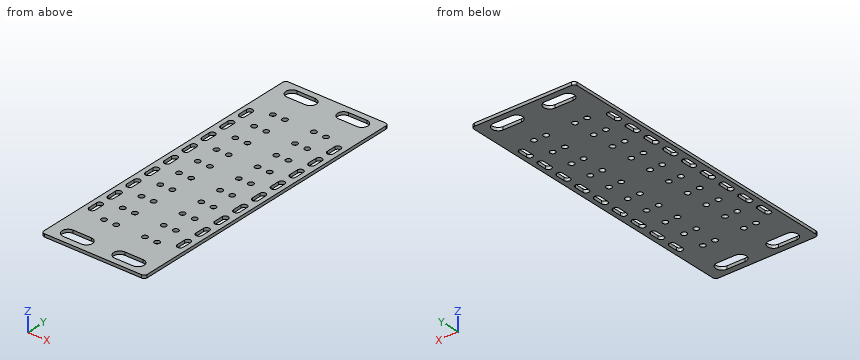
```python
from build123d import *

# Parameters (mm, degrees)
ESBO_O1_W             = 68
ESBO_O1_H             = 195
FLANGE_BASE1_DEPTH    = 2
FILETE1_R             = 2
ESBO_O2_R             = 1.75
CORTE_EXTRUS_O1_DEPTH = 10


# Sheet-metal steps are written as plain solids
with BuildPart() as part:
    # Esboço1 → Flange-base1 (new body)
    with BuildSketch(Plane.XY):
        with Locations((34, 97.5)):
            Rectangle(ESBO_O1_W, ESBO_O1_H)
    extrude(amount=-FLANGE_BASE1_DEPTH)

    # Filete1
    filete1_edges = [part.edges().sort_by_distance(p)[0] for p in [
        (0, 195, -1),
        (68, 195, -1),
        (68, 0, -1),
        (0, 0, -1),
    ]]
    fillet(filete1_edges, radius=FILETE1_R)

    # Esboço2 → Corte-extrusão1 (cut)
    with BuildSketch(Plane.XY):
        with Locations((16.5, 165)):
            Circle(ESBO_O2_R)
        with Locations((24.5, 165)):
            Circle(ESBO_O2_R)
        with Locations((43.5, 165)):
            Circle(ESBO_O2_R)
        with Locations((51.5, 165)):
            Circle(ESBO_O2_R)
        with Locations((43.5, 150)):
            Circle(ESBO_O2_R)
        with Locations((51.5, 150)):
            Circle(ESBO_O2_R)
        with Locations((43.5, 135)):
            Circle(ESBO_O2_R)
        with Locations((51.5, 135)):
            Circle(ESBO_O2_R)
        with Locations((43.5, 120)):
            Circle(ESBO_O2_R)
        with Locations((51.5, 120)):
            Circle(ESBO_O2_R)
        with Locations((43.5, 105)):
            Circle(ESBO_O2_R)
        with Locations((51.5, 105)):
            Circle(ESBO_O2_R)
        with Locations((16.5, 150)):
            Circle(ESBO_O2_R)
        with Locations((24.5, 150)):
            Circle(ESBO_O2_R)
        with Locations((16.5, 135)):
            Circle(ESBO_O2_R)
        with Locations((24.5, 135)):
            Circle(ESBO_O2_R)
        with Locations((16.5, 120)):
            Circle(ESBO_O2_R)
        with Locations((24.5, 120)):
            Circle(ESBO_O2_R)
        with Locations((16.5, 105)):
            Circle(ESBO_O2_R)
        with Locations((24.5, 105)):
            Circle(ESBO_O2_R)
        with Locations((16.5, 90)):
            Circle(ESBO_O2_R)
        with Locations((24.5, 90)):
            Circle(ESBO_O2_R)
        with Locations((43.5, 90)):
            Circle(ESBO_O2_R)
        with Locations((51.5, 90)):
            Circle(ESBO_O2_R)
        with Locations((16.5, 75)):
            Circle(ESBO_O2_R)
        with Locations((24.5, 75)):
            Circle(ESBO_O2_R)
        with Locations((43.5, 75)):
            Circle(ESBO_O2_R)
        with Locations((51.5, 75)):
            Circle(ESBO_O2_R)
        with Locations((16.5, 60)):
            Circle(ESBO_O2_R)
        with Locations((24.5, 60)):
            Circle(ESBO_O2_R)
        with Locations((43.5, 60)):
            Circle(ESBO_O2_R)
        with Locations((51.5, 60)):
            Circle(ESBO_O2_R)
        with Locations((16.5, 45)):
            Circle(ESBO_O2_R)
        with Locations((24.5, 45)):
            Circle(ESBO_O2_R)
        with Locations((43.5, 45)):
            Circle(ESBO_O2_R)
        with Locations((51.5, 45)):
            Circle(ESBO_O2_R)
        with Locations((16.5, 30)):
            Circle(ESBO_O2_R)
        with Locations((24.5, 30)):
            Circle(ESBO_O2_R)
        with Locations((43.5, 30)):
            Circle(ESBO_O2_R)
        with Locations((51.5, 30)):
            Circle(ESBO_O2_R)
        with BuildLine():
            Line((11, 191), (23, 191))
            ThreePointArc((23, 191), (27, 187), (23, 183))
            Line((23, 183), (11, 183))
            ThreePointArc((11, 183), (7, 187), (11, 191))
        make_face()
        with BuildLine():
            Line((57, 191), (45, 191))
            ThreePointArc((45, 191), (41, 187), (45, 183))
            Line((45, 183), (57, 183))
            ThreePointArc((57, 183), (61, 187), (57, 191))
        make_face()
        with BuildLine():
            Line((11, 4), (23, 4))
            ThreePointArc((23, 4), (27, 8), (23, 12))
            Line((23, 12), (11, 12))
            ThreePointArc((11, 12), (7, 8), (11, 4))
        make_face()
        with BuildLine():
            Line((57, 4), (45, 4))
            ThreePointArc((45, 4), (41, 8), (45, 12))
            Line((45, 12), (57, 12))
            ThreePointArc((57, 12), (61, 8), (57, 4))
        make_face()
        with BuildLine():
            Line((7, 160.5), (7, 154.5))
            ThreePointArc((7, 154.5), (5, 152.5), (3, 154.5))
            Line((3, 154.5), (3, 160.5))
            ThreePointArc((3, 160.5), (5, 162.5), (7, 160.5))
        make_face()
        with BuildLine():
            Line((65, 160.5), (65, 154.5))
            ThreePointArc((65, 154.5), (63, 152.5), (61, 154.5))
            Line((61, 154.5), (61, 160.5))
            ThreePointArc((61, 160.5), (63, 162.5), (65, 160.5))
        make_face()
        with BuildLine():
            Line((65, 145.5), (65, 139.5))
            ThreePointArc((65, 139.5), (63, 137.5), (61, 139.5))
            Line((61, 139.5), (61, 145.5))
            ThreePointArc((61, 145.5), (63, 147.5), (65, 145.5))
        make_face()
        with BuildLine():
            Line((65, 130.5), (65, 124.5))
            ThreePointArc((65, 124.5), (63, 122.5), (61, 124.5))
            Line((61, 124.5), (61, 130.5))
            ThreePointArc((61, 130.5), (63, 132.5), (65, 130.5))
        make_face()
        with BuildLine():
            Line((65, 115.5), (65, 109.5))
            ThreePointArc((65, 109.5), (63, 107.5), (61, 109.5))
            Line((61, 109.5), (61, 115.5))
            ThreePointArc((61, 115.5), (63, 117.5), (65, 115.5))
        make_face()
        with BuildLine():
            Line((65, 100.5), (65, 94.5))
            ThreePointArc((65, 94.5), (63, 92.5), (61, 94.5))
            Line((61, 94.5), (61, 100.5))
            ThreePointArc((61, 100.5), (63, 102.5), (65, 100.5))
        make_face()
        with BuildLine():
            Line((65, 85.5), (65, 79.5))
            ThreePointArc((65, 79.5), (63, 77.5), (61, 79.5))
            Line((61, 79.5), (61, 85.5))
            ThreePointArc((61, 85.5), (63, 87.5), (65, 85.5))
        make_face()
        with BuildLine():
            Line((65, 70.5), (65, 64.5))
            ThreePointArc((65, 64.5), (63, 62.5), (61, 64.5))
            Line((61, 64.5), (61, 70.5))
            ThreePointArc((61, 70.5), (63, 72.5), (65, 70.5))
        make_face()
        with BuildLine():
            Line((65, 55.5), (65, 49.5))
            ThreePointArc((65, 49.5), (63, 47.5), (61, 49.5))
            Line((61, 49.5), (61, 55.5))
            ThreePointArc((61, 55.5), (63, 57.5), (65, 55.5))
        make_face()
        with BuildLine():
            Line((7, 145.5), (7, 139.5))
            ThreePointArc((7, 139.5), (5, 137.5), (3, 139.5))
            Line((3, 139.5), (3, 145.5))
            ThreePointArc((3, 145.5), (5, 147.5), (7, 145.5))
        make_face()
        with BuildLine():
            Line((7, 130.5), (7, 124.5))
            ThreePointArc((7, 124.5), (5, 122.5), (3, 124.5))
            Line((3, 124.5), (3, 130.5))
            ThreePointArc((3, 130.5), (5, 132.5), (7, 130.5))
        make_face()
        with BuildLine():
            Line((7, 115.5), (7, 109.5))
            ThreePointArc((7, 109.5), (5, 107.5), (3, 109.5))
            Line((3, 109.5), (3, 115.5))
            ThreePointArc((3, 115.5), (5, 117.5), (7, 115.5))
        make_face()
        with BuildLine():
            Line((7, 100.5), (7, 94.5))
            ThreePointArc((7, 94.5), (5, 92.5), (3, 94.5))
            Line((3, 94.5), (3, 100.5))
            ThreePointArc((3, 100.5), (5, 102.5), (7, 100.5))
        make_face()
        with BuildLine():
            Line((7, 85.5), (7, 79.5))
            ThreePointArc((7, 79.5), (5, 77.5), (3, 79.5))
            Line((3, 79.5), (3, 85.5))
            ThreePointArc((3, 85.5), (5, 87.5), (7, 85.5))
        make_face()
        with BuildLine():
            Line((7, 70.5), (7, 64.5))
            ThreePointArc((7, 64.5), (5, 62.5), (3, 64.5))
            Line((3, 64.5), (3, 70.5))
            ThreePointArc((3, 70.5), (5, 72.5), (7, 70.5))
        make_face()
        with BuildLine():
            Line((7, 55.5), (7, 49.5))
            ThreePointArc((7, 49.5), (5, 47.5), (3, 49.5))
            Line((3, 49.5), (3, 55.5))
            ThreePointArc((3, 55.5), (5, 57.5), (7, 55.5))
        make_face()
        with BuildLine():
            Line((7, 40.5), (7, 34.5))
            ThreePointArc((7, 34.5), (5, 32.5), (3, 34.5))
            Line((3, 34.5), (3, 40.5))
            ThreePointArc((3, 40.5), (5, 42.5), (7, 40.5))
        make_face()
        with BuildLine():
            Line((65, 40.5), (65, 34.5))
            ThreePointArc((65, 34.5), (63, 32.5), (61, 34.5))
            Line((61, 34.5), (61, 40.5))
            ThreePointArc((61, 40.5), (63, 42.5), (65, 40.5))
        make_face()
    extrude(amount=-CORTE_EXTRUS_O1_DEPTH, mode=Mode.SUBTRACT)


solid = part.part
```
The listing builds one solid part. Answer for the finished solid, in the listing's coordinates (mm). Give positions to 0.01 mm unless a question says otherwise; leave off trailing zeros. Order: outer loops, then holes, each group sorted by start corner. A loop starts at its lowest first (then second) coordinate and runs counter-clockwise, first axis right, second up. Notation, with made-up numbers: (41.5, -14.5) -> (78.5, -14.5) arc R28 cw to (78.5, 4.5) -> close; hole circle Ø6 at (10, 40.5). An arc over 180 degrees is marked (long way). Answer as a JSON object with one key per item and string values. Group by question number.
Item 1: The part is cut by section C-C on y = 135. Write down the section's boundary in (x, z).
Item 2: A flat-ended cylindrical pin translates along its axis: pin 1 (5.5 mm diameter, centred on x = 43.5, y = 165, fed in from -Z). Find the tip coordinate at first contact, or state that the pin passes through.
Item 3: Consider L1, parallel to X at y = 125.5, z = -0.55; L2, parallel to X at y = 165, z = -1.15; L3, parallel to Y at x = 20.5, z = -1. Determine where each line is inside the solid, lowest interval first. Write a range as from..to.
Item 4: The part is cut by section D-D on x = 63. Give the number of separate pieces and of enclosed holes in the cut face, and give its area (3 significant figures).
Item 5: The part is cut by section A-A on y = 111.5. Write down the section's boundary in (x, z), and give its area (3 significant figures).
Item 6: The part is cut by section B-B on x = 48. Write down the section's boundary in (y, z), and give its area (3 significant figures).
Result set:
{
 "1": {"outline": "(0, -2) -> (14.75, -2) -> (14.75, 0) -> (0, 0) -> close; (18.25, -2) -> (22.75, -2) -> (22.75, 0) -> (18.25, 0) -> close; (26.25, -2) -> (41.75, -2) -> (41.75, 0) -> (26.25, 0) -> close; (45.25, -2) -> (49.75, -2) -> (49.75, 0) -> (45.25, 0) -> close; (53.25, -2) -> (68, -2) -> (68, 0) -> (53.25, 0) -> close"},
 "2": {"pin 1": "z = -2"},
 "3": {"L1": "0..3, 7..61, 65..68", "L2": "0..14.75, 18.25..22.75, 26.25..41.75, 45.25..49.75, 53.25..68", "L3": "0..4, 12..183, 191..195"},
 "4": {"separate pieces": "10", "enclosed holes": "0", "area": "210 mm²"},
 "5": {"outline": "(0, -2) -> (3, -2) -> (3, 0) -> (0, 0) -> close; (7, -2) -> (61, -2) -> (61, 0) -> (7, 0) -> close; (65, -2) -> (68, -2) -> (68, 0) -> (65, 0) -> close", "area": "120 mm²"},
 "6": {"outline": "(0, -2) -> (4, -2) -> (4, 0) -> (0, 0) -> close; (12, -2) -> (183, -2) -> (183, 0) -> (12, 0) -> close; (191, -2) -> (195, -2) -> (195, 0) -> (191, 0) -> close", "area": "358 mm²"}
}
